Read the model definition and answer for the solid it produces. Units are mm, in the model's axes. Coordinates: 2 decimals unless noted, no trailing zeros. Loops run counter-clockwise (first coordinate to the right, second up) from the corner with the lowest first, then second, coordinate; pieces in that order, holes last.
Autodesk Inventor part; units mm, degrees
ref_plane "YZ Plane" through (0, 0, 0) normal (1, 0, 0) x (0, 1, 0)
ref_plane "XZ Plane" through (0, 0, 0) normal (0, 1, 0) x (-1, 0, 0)
ref_plane "XY Plane" through (0, 0, 0) normal (0, 0, 1) x (1, 0, 0)
sketch "Эскиз1" plane through (0, 0, 0) normal (0, 1, 0) x (-1, 0, 0)
  circle A0 centre (0, 0) radius 2
  dimension "d0" = 4
extrude "Выдавливание1" add sketch "Эскиз1" along normal blind 6.75
sketch "Эскиз2" plane through (0, 0, 0) normal (0, -1, 0) x (1, 0, 0)
  circle A0 centre (0, 0) radius 2
  circle A1 centre (0, 0) radius 1.5 construction
  line L0 (0, 1.5) -> (1.299, 0.75)
  line L1 (1.299, 0.75) -> (1.299, -0.75)
  line L2 (1.299, -0.75) -> (0, -1.5)
  line L3 (0, -1.5) -> (-1.299, -0.75)
  line L4 (-1.299, -0.75) -> (-1.299, 0.75)
  line L5 (-1.299, 0.75) -> (0, 1.5)
  dimension "d3" = 3
extrude "Выдавливание2" cut sketch "Эскиз2" against normal blind 1.25 contours L0 L1 L2 L3 L4 L5
fillet "Сопряжение1" radius 0.25 1 edges at (2, 0, 0)
thread "Резьба1"
properties part number "Bolt"
Item 1: A cutting plane is placed at B-B on y = 3.5. Determine the outline of the cut face in (x, z).
Numbers:
outline: circle Ø4 at (0, 0)
Item 2: A cutting plane is placed at A-A on z = 0. Determine the outline of the cut face in (x, y), then the cut area to 3 significant figures.
Numbers:
outline: (-2, 0.25) arc R0.25 ccw to (-1.75, 0) - (-1.3, 0) - (-1.3, 1.25) - (1.3, 1.25) - (1.3, 0) - (1.75, 0) arc R0.25 ccw to (2, 0.25) - (2, 6.75) - (-2, 6.75) - close
area: 23.7 mm2
Item 3: Find the intervals of material crossed by line 1 along Y through (x, z) = (-0.15, 1.15); line 2 along X through (y, z) = (6, 0.1); line 3 along Y through (x, z) = (-0.55, 1.7), in increasing order.
Numbers:
line 1: y = 1.25 to 6.75
line 2: x = -2 to 2
line 3: y = 0 to 6.75
Item 4: Determine the mould class of faces 1 (the face through (-1.299, 1, 0)), 2 (the face through (0, 6.75, 0)), 3 (the face through (0, 3, 2)) for opening direction Z: released by +Z, released by -Z, zero draft, split by the parting line, or undercut.
Numbers:
face 1: undercut
face 2: zero draft
face 3: split by the parting line
Item 5: Given pin 1 (0.8 mm diameter, centred on x = -0.5, z = 0.5, fed in from -Y); pin 2 (2 mm diameter, centred on y = 3.5, z = -1.5, fed in from +X), each flat-ended and moving along its own axis, determine where each tip first touches the part or whether it passes through.
Numbers:
pin 1: stops at y = 1.25
pin 2: stops at x = 1.94
